The listing builds one solid part. Answer for the finished solid, in the listing's coordinates (mm). A direction names the side the tool comes from. Give positions to 0.01 mm unless a question says otherwise; leave off trailing zeros. Write each loop counter-clockwise with the first axis right and the second up, starting at its lowest first coordinate (ties: lowest second). Pieces come first, ordered by that corner, then holes. Notation, with made-up numbers: (70, 23.25) - (94, 23.25) arc R36 cw to (94, 58.25) - close; hole circle Ø9 at (81, 5). An arc over 180 degrees is marked (long way). Use a Markdown table: item, result. Add a question column.
from build123d import *

# Parameters (mm, degrees)
BOSS_EXTRUDE4_DEPTH          = 70
BOSS_EXTRU_5_DEPTH           = 55.5
BOSS_EXTRU_5_DEPTH_BACK      = 55.5
ENL_V_MAT_EXTRU_3_DEPTH      = 35.5
ENL_V_MAT_EXTRU_3_DEPTH_BACK = 35.5
BOSS_EXTRU_3_REACH           = 156.068
ESQUISSE9_W                  = 5
ESQUISSE9_H                  = 247.389280508
ESQUISSE8_R                  = 1
ENL_V_MAT_EXTRU_1_DEPTH      = 156.154173773
ENL_V_MAT_EXTRU_1_DEPTH_BACK = 156.154173773
ESQUISSE17_W                 = 130
ESQUISSE17_H                 = 7.5
ENL_V_MAT_EXTRU_2_DEPTH      = 154.81098023
ENL_V_MAT_EXTRU_2_DEPTH_BACK = 154.81098023
ESQUISSE19_R                 = 3.5
ENL_V_MAT_EXTRU_4_DEPTH      = 194.385153616


with BuildPart() as part:
    # Sketch4 → Boss-Extrude4 (new, symmetric)
    with BuildSketch(Plane(origin=(0, 0, 0), x_dir=(0, 0, -1), z_dir=(1, 0, 0))):
        with BuildLine():
            Line((0, 0), (87.331538291, 0))
            ThreePointArc((87.331538291, 0), (95.783903526, 1.873844259), (102.652427153, 7.144247806))
            Line((102.652427153, 7.144247806), (130.821150271, 40.714424781))
            ThreePointArc((130.821150271, 40.714424781), (131.101676959, 42.845236523), (129.289061385, 44))
            Line((129.289061385, 44), (127.051038779, 44))
            Line((127.051038779, 44), (100.320888862, 12.144247806))
            ThreePointArc((100.320888862, 12.144247806), (93.452365235, 6.873844259), (85, 5))
            Line((85, 5), (0, 5))
            Line((0, 5), (0, 0))
        make_face()
    boss_extrude4 = extrude(amount=BOSS_EXTRUDE4_DEPTH, both=True)

    # Esquisse15 → Boss.-Extru.5 (add, two sides)
    with BuildSketch(Plane(origin=(0, 0, 0), x_dir=(0, 0, -1), z_dir=(1, 0, 0))) as boss_extru_5_sk:
        with BuildLine():
            Line((100.320888862, 12.144247806), (110.47494439, 24.245379961))
            ThreePointArc((110.47494439, 24.245379961), (106.073337597, 24.643477634), (103.138451771, 27.94787914))
            Line((103.138451771, 27.94787914), (99.337028752, 15.589829192))
            ThreePointArc((99.337028752, 15.589829192), (93.911998594, 7.934500381), (85, 5))
            ThreePointArc((85, 5), (93.452365235, 6.873844259), (100.320888862, 12.144247806))
        make_face()
    extrude(amount=BOSS_EXTRU_5_DEPTH)
    extrude(boss_extru_5_sk.sketch, amount=-BOSS_EXTRU_5_DEPTH_BACK)

    # Esquisse18 → Enlèv. mat.-Extru.3 (cut, two sides)
    with BuildSketch(Plane(origin=(0, 0, 0), x_dir=(0, 0, -1), z_dir=(1, 0, 0))) as enl_v_mat_extru_3_sk:
        with BuildLine():
            Line((100.320888862, 12.144247806), (110.47494439, 24.245379961))
            ThreePointArc((110.47494439, 24.245379961), (106.073337597, 24.643477634), (103.138451771, 27.94787914))
            Line((103.138451771, 27.94787914), (99.337028752, 15.589829192))
            ThreePointArc((99.337028752, 15.589829192), (93.911998594, 7.934500381), (85, 5))
            ThreePointArc((85, 5), (93.452365235, 6.873844259), (100.320888862, 12.144247806))
        make_face()
    extrude(amount=ENL_V_MAT_EXTRU_3_DEPTH, mode=Mode.SUBTRACT)
    extrude(enl_v_mat_extru_3_sk.sketch, amount=-ENL_V_MAT_EXTRU_3_DEPTH_BACK, mode=Mode.SUBTRACT)

    # Mirror2: Boss-Extrude4 across plane
    add(boss_extrude4.mirror(Plane(origin=(70, 5, 0), x_dir=(1, 0, 0), z_dir=(0, 0, -1))))

    # Esquisse9 → Boss.-Extru.3 (add, up to next)
    with BuildSketch(Plane(origin=(0, 40, 0), x_dir=(1, 0, 0), z_dir=(0, 1, 0)), mode=Mode.PRIVATE) as boss_extru_3_sk1:
        with Locations((67.5, 0)):
            Rectangle(ESQUISSE9_W, ESQUISSE9_H)
    boss_extru_3_tool1 = extrude(boss_extru_3_sk1.sketch, amount=-BOSS_EXTRU_3_REACH, mode=Mode.PRIVATE) - part.part
    # Esquisse9 → Boss.-Extru.3 (add, up to next)
    with BuildSketch(Plane(origin=(0, 40, 0), x_dir=(1, 0, 0), z_dir=(0, 1, 0)), mode=Mode.PRIVATE) as boss_extru_3_sk2:
        with Locations((-67.5, 0)):
            Rectangle(ESQUISSE9_W, ESQUISSE9_H)
    boss_extru_3_tool2 = extrude(boss_extru_3_sk2.sketch, amount=-BOSS_EXTRU_3_REACH, mode=Mode.PRIVATE) - part.part
    add(boss_extru_3_tool1.solids().sort_by_distance((67.5, 40, 0))[0])
    add(boss_extru_3_tool2.solids().sort_by_distance((-67.5, 40, 0))[0])

    # Esquisse8 → Enlèv. mat.-Extru.1 (cut, two sides)
    with BuildSketch(Plane(origin=(0, 0, 0), x_dir=(0, 0, -1), z_dir=(1, 0, 0))) as enl_v_mat_extru_1_sk:
        with Locations((0, 20)):
            Circle(ESQUISSE8_R)
        with Locations((60, 20)):
            Circle(ESQUISSE8_R)
        with Locations((-60, 20)):
            Circle(ESQUISSE8_R)
    extrude(amount=ENL_V_MAT_EXTRU_1_DEPTH, mode=Mode.SUBTRACT)
    extrude(enl_v_mat_extru_1_sk.sketch, amount=-ENL_V_MAT_EXTRU_1_DEPTH_BACK, mode=Mode.SUBTRACT)

    # Esquisse17 → Enlèv. mat.-Extru.2 (cut, two sides)
    with BuildSketch(Plane(origin=(0, 5, 0), x_dir=(1, 0, 0), z_dir=(0, 1, 0))) as enl_v_mat_extru_2_sk:
        Rectangle(ESQUISSE17_W, ESQUISSE17_H)
        with Locations((0, 15)):
            Rectangle(ESQUISSE17_W, ESQUISSE17_H)
        with Locations((0, 30)):
            Rectangle(ESQUISSE17_W, ESQUISSE17_H)
        with Locations((0, 45)):
            Rectangle(ESQUISSE17_W, ESQUISSE17_H)
        with Locations((0, 60)):
            Rectangle(ESQUISSE17_W, ESQUISSE17_H)
        with Locations((0, 75)):
            Rectangle(ESQUISSE17_W, ESQUISSE17_H)
        with Locations((0, -15)):
            Rectangle(ESQUISSE17_W, ESQUISSE17_H)
        with Locations((0, -30)):
            Rectangle(ESQUISSE17_W, ESQUISSE17_H)
        with Locations((0, -45)):
            Rectangle(ESQUISSE17_W, ESQUISSE17_H)
        with Locations((0, -60)):
            Rectangle(ESQUISSE17_W, ESQUISSE17_H)
        with Locations((0, -75)):
            Rectangle(ESQUISSE17_W, ESQUISSE17_H)
    extrude(amount=ENL_V_MAT_EXTRU_2_DEPTH, mode=Mode.SUBTRACT)
    extrude(enl_v_mat_extru_2_sk.sketch, amount=-ENL_V_MAT_EXTRU_2_DEPTH_BACK, mode=Mode.SUBTRACT)

    # Esquisse19 → Enlèv. mat.-Extru.4 (cut, symmetric)
    with BuildSketch(Plane(origin=(-65, 0, 0), x_dir=(0, 0, -1), z_dir=(1, 0, 0))):
        with Locations((108.777551806, 30.001125385)):
            Circle(ESQUISSE19_R)
    enl_v_mat_extru_4 = extrude(amount=ENL_V_MAT_EXTRU_4_DEPTH, both=True, mode=Mode.SUBTRACT)

    # Symétrie1: Enlèv. mat.-Extru.4 across plane
    add(enl_v_mat_extru_4.mirror(Plane.XY), mode=Mode.SUBTRACT)


solid = part.part
1. The part is cut by section A-A (z = -7.5). Give the vertices of the cut face in (x, y).
2. Consider L1, parallel to X at y = 32.5, z = 36.5; L2, parallel to Y at x = 68.55, z = 0; L3, parallel to Y at x = -1.5, z = 34.5. Determine where each line is inside the solid, lowest interval first. Write a range as [from, to].
3. The part is cut by section B-B (x = 60). Count the separate pieces of the cut face and the enclosed holes in it, and give its area (3 significant figures).
4. Given P1, Ø4, axis at x = -1, y = 2, coming from the -Z side; P2, Ø8, axis at x = -20.5, z = 22, coming from the +Y side; P3, Ø4, axis at x = -23, y = 2.5, coming from the -Z side, each flat-ended and moving along its own axis, determine where each tip first touches the part or whether it passes through.
5. Which of the six approach directions +Z, -Z, +X, -X, +Y, -Y give full straight-line access (tool end or side, diameter ignored) to faces 1 (the flat face through (-68, 40, -2)), 2 (the flat face through (-1, 3, 3.75)), 3 (the cylindrical face through (-45, 8, -94))?
6. For a pull along X with two mould halves and no side action, classify faces 4 (the flat face through (-1, 3, -63.75)), 5 (the cylindrical face through (0.98, 1.82, -95.67)) as released by +X, released by -X, zero draft, split by the parting line, or undercut.
Check values:
| question | item | result |
|---|---|---|
| 1 | outline | (-70, 0) - (70, 0) - (70, 40) - (65, 40) - (65, 5) - (-65, 5) - (-65, 40) - (-70, 40) - close |
| 2 | L1 | x = [-70, -65], [65, 70] |
| 2 | L2 | y = [0, 19], [21, 40] |
| 2 | L3 | y = [0, 5] |
| 3 | separate pieces | 12 |
| 3 | enclosed holes | 0 |
| 3 | area | 1,080 mm2 |
| 4 | P1 | stops at z = -99.33 |
| 4 | P2 | stops at y = 5 |
| 4 | P3 | stops at z = -99.97 |
| 5 | face 1 | +X, -X, +Y |
| 5 | face 2 | +Y, -Y |
| 5 | face 3 | +Y |
| 6 | face 4 | undercut |
| 6 | face 5 | zero draft |
